from build123d import *

# Parameters (mm, degrees)
BOSS_EXTRUDE1_DEPTH = 10
BOSS_EXTRUDE2_DEPTH = 15


with BuildPart() as part:
    # Sketch1 → Boss-Extrude1 (new body)
    with BuildSketch(Plane.XY):
        Polygon((0, 0), (0, 25), (-30, 0), align=None)
    extrude(amount=BOSS_EXTRUDE1_DEPTH)

    # Sketch2 → Boss-Extrude2 (add)
    with BuildSketch(Plane.XY.offset(10)):
        Polygon((-30, 25), (0, 25), (0, 5), align=None)
    extrude(amount=BOSS_EXTRUDE2_DEPTH)


solid = part.part
Here's how the part is built. I have some questions about the finished solid (model axes, mm). A direction names the side the tool comes from. Give positions to 0.01 mm unless a question says otherwise; leave off trailing zeros. Order: outer loops, then holes, each group sorted by start corner. A loop starts at its lowest first (then second) coordinate and runs counter-clockwise, first axis right, second up. Notation, with made-up numbers: (-35.5, 39) -> (-9.5, 39) arc R15 cw to (-9.5, 56) -> close; hole circle Ø2 at (42.25, 75.5). An arc over 180 degrees is marked (long way). One line per item, written item: value. Start each with the question number.
1. For faces 1 (the face through (-15, 25, 17)), 2 (the face through (-14.79, 12.675, 4.93)), 3 (the face through (-15, 15, 17)), which set-ups out of +Z, -Z, +X, -X, +Y, -Y let a thin tool reach every point of the face, with its end or its side?
2. Imagine slicing it at B-B, the plane y = 20.5. List the corners of the cut face in (x, z) for me.
3. Imagine slicing it at A-A, the plane x = -15. List the corners of the cut face in (y, z) for me.
4. I need wall thicknesses on probe 1 along Z at (x, y) = (-17, 21.5); probe 2 along Z at (x, y) = (-9, 10.25); probe 3 along Y at (x, z) = (-15.25, 20.5). Which ranges of each line are inside material? Lowest first, please. Write a range as from..to.
5. Imagine slicing it at C-C, the plane z = 15.5. List the corners of the cut face in (x, y) for me.
6. Will these pins go through, and if not, where does the flat tip stop? pin 1 Ø7 at (x, y) = (-21.5, 8) entering from +Z; pin 2 Ø3 at (y, z) = (16.5, 13.5) entering from -X; pin 3 Ø1 at (x, z) = (-12.5, 11) entering from -Y.
7. Imagine slicing it at D-D, the plane x = -22. List the corners of the cut face in (y, z) for me, plus the area to 3 significant figures.
Values follow:
1. face 1: +Z, -Z, +X, -X, +Y
1. face 2: -Z, -X, +Y
1. face 3: +Z, -X, -Y
2. outline: (-23.25, 10) -> (-5.4, 10) -> (-5.4, 0) -> (0, 0) -> (0, 25) -> (-23.25, 25) -> close
3. outline: (0, 0) -> (12.5, 0) -> (12.5, 10) -> (0, 10) -> close; (15, 10) -> (25, 10) -> (25, 25) -> (15, 25) -> close
4. probe 1: z = 10..25
4. probe 2: z = 0..10
4. probe 3: y = 15.17..25
5. outline: (-30, 25) -> (0, 5) -> (0, 25) -> close
6. pin 1: stops at z = 10
6. pin 2: stops at x = -19.5
6. pin 3: stops at y = 13
7. outline: (0, 0) -> (6.67, 0) -> (6.67, 10) -> (0, 10) -> close; (19.67, 10) -> (25, 10) -> (25, 25) -> (19.67, 25) -> close
7. area: 147 mm2
